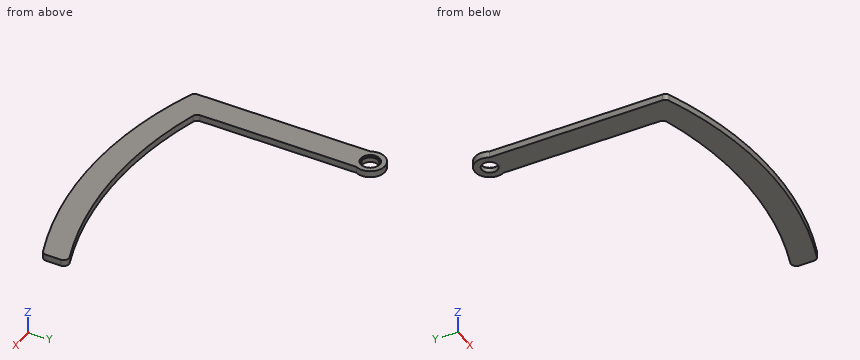
Autodesk Inventor part; units mm, degrees
ref_plane "YZ Plane" through (0, 0, 0) normal (1, 0, 0) x (0, 1, 0)
ref_plane "XZ Plane" through (0, 0, 0) normal (0, 1, 0) x (-1, 0, 0)
ref_plane "XY Plane" through (0, 0, 0) normal (0, 0, 1) x (1, 0, 0)
sketch "スケッチ1" plane through (0, 0, 0) normal (0, 0, 1) x (1, 0, 0)
  line L0 (-5, -38) -> (5, -38)
  line L1 (5, -38) -> (5, 38)
  line L2 (5, 38) -> (-5, 38)
  line L3 (-5, 38) -> (-5, -38)
  line L4 (-5, -38) -> (5, 38) construction
  line L5 (5, -38) -> (-5, 38) construction
  line L6 (-5, -38) -> (100, -38)
  line L7 (100, -38) -> (100, -28)
  line L8 (100, -28) -> (-5, -28)
  line L9 (-5, -28) -> (-5, -38)
  line L10 (47.5, -38) -> (47.5, -48)
  arc A0 (-5, -28) -> (100, -28) centre (47.5, 104.8125) ccw
  arc A1 (-5, -38) -> (100, -38) centre (47.5, 94.8125) ccw
  point P0 (0, 0)
  point P1 (5, -31.5296)
  dimension "d0" = 10
  dimension "d1" = 76
  dimension "d2" = 105
  dimension "d3" = 10
  dimension "d4" = 10
extrude "押し出し1" add sketch "スケッチ1" along normal mid plane 2.5 contours L3 A0 L1 L0 | L0 L6 L10 A1 | L1 A0 L6 | L3 L2 L1 L8 | L8 L1 A0 | L10 L6 A1 | A0 L7 L6 picked at (-0.5654, -28.4196)
sketch "スケッチ2" plane through (0, 0, 1.25) normal (0, 0, 1) x (1, 0, 0)
  line L0 (5, 38) -> (-5, 38)
  line L1 (5, -31.5296) -> (5, 38)
  circle A0 centre (0, 33) radius 3.05
  circle A1 centre (0, 33) radius 3.65
  point P0 (0, 0)
  dimension "d7" = 5
  dimension "d8" = 5
  dimension "d9" = 6.1
  dimension "d10" = 7.3
extrude "押し出し2" cut sketch "スケッチ2" against normal blind 0.6 contours A0 | A1
sketch "スケッチ3" plane through (0, 33, 0.65) normal (0, 0, 1) x (1, 0, 0)
  circle A0 centre (0, 0) radius 3.05
  point P0 (0, -33)
  dimension "d13" = 6.1
extrude "押し出し3" cut sketch "スケッチ3" against normal blind 1.9
sketch "スケッチ6" plane through (0, 0, 1.25) normal (0, 0, 1) x (1, 0, 0)
  circle A0 centre (0, 33) radius 3.65
  line L0 (-5, 38) -> (-5, -38)
  arc A1 (-5, -38) -> (100, -38) centre (47.5, 94.8125) ccw
  line L1 (100, -38) -> (100, -28)
  arc A2 (5, -31.5296) -> (100, -28) centre (47.5, 104.8125) ccw
  line L2 (5, -31.5296) -> (5, 38)
  line L3 (5, 38) -> (-5, 38)
  circle A3 centre (0, 33) radius 5.65
  point P0 (0, 0)
  point P1 (-5, 30.3689)
  point P2 (-5, 35.6311)
  point P3 (-2.6311, 38)
  point P4 (2.6311, 38)
  point P5 (5, 35.6311)
  point P6 (5, 30.3689)
  dimension "d18" = 11.3
extrude "押し出し5" add sketch "スケッチ6" against normal blind 2.5 contours L0 A3 | A3 L3 | L2 A3
sketch "スケッチ7" plane through (0, 0, 1.25) normal (0, 0, 1) x (1, 0, 0)
  circle A0 centre (0, 33) radius 3.65
  line L0 (-5, 38) -> (-5, 35.6311)
  arc A1 (-5, 35.6311) -> (-5, 30.3689) centre (0, 33) ccw
  line L1 (-5, 30.3689) -> (-5, -38)
  arc A2 (-5, -38) -> (100, -38) centre (47.5, 94.8125) ccw
  line L2 (100, -38) -> (100, -28)
  arc A3 (5, -31.5296) -> (100, -28) centre (47.5, 104.8125) ccw
  line L3 (5, -31.5296) -> (5, 30.3689)
  arc A4 (5, 30.3689) -> (5, 35.6311) centre (0, 33) ccw
  line L4 (5, 35.6311) -> (5, 38)
  line L5 (5, 38) -> (2.6311, 38)
  arc A5 (2.6311, 38) -> (-2.6311, 38) centre (0, 33) ccw
  line L6 (-2.6311, 38) -> (-5, 38)
  circle A6 centre (0, 33) radius 5.65
  point P0 (0, 0)
  point P1 (-5, 35.6311)
  point P2 (-2.6311, 38)
  point P3 (2.6311, 38)
  point P4 (5, 35.6311)
extrude "押し出し6" cut sketch "スケッチ7" against normal blind 2.5 contours L6 A6 L0 | L5 L4 A6
fillet "フィレット1" radius 2 4 edges at (-5, -38, 0) (5, -31.5296, 0) (100, -28, 0) (100, -38, 0)
properties part number "指_大"
Read the model definition and answer for the solid it produces. Units are mm, in the model's axes. Round coordinates to 2 decimals unless told otherwise and drop trailing zeros. Write each loop counter-clockwise with the first axis right and the second up, starting at its lowest first coordinate (ties: lowest second). Pieces come first, ordered by that corner, then holes. Notation, with made-up numbers: (67.5, 31) - (105.5, 31) arc R28 cw to (105.5, 49) - close; hole circle Ø1 at (82.25, 47). An arc over 180 degrees is marked (long way). One line per item, written item: value.
Q1. Find section C-C (x = 0). Determine the outline of the cut face in (y, z).
The answers:
outline: (-39.87, -1.25) - (29.95, -1.25) - (29.95, 0.65) - (29.35, 0.65) - (29.35, 1.25) - (-39.87, 1.25) - close; (36.05, -1.25) - (38.65, -1.25) - (38.65, 1.25) - (36.65, 1.25) - (36.65, 0.65) - (36.05, 0.65) - close
Q2. Each of these flat-tipped pins is pushed along its axis until it touches: P1, Ø1.2, axis at y = 8.5, z = -0.5, coming from the -X side; P2, Ø1.2, axis at y = 10.5, z = 0, coming from the +X side; P3, Ø6.5, axis at x = 0, y = 33, coming from the +Z side. Where does it stop, or does it pass through?
The answers:
P1: stops at x = -5
P2: stops at x = 5
P3: stops at z = 0.65
Q3. Find section D-D (y = 9). Determine the outline of the cut face in (x, z), and give its area (3 significant figures).
The answers:
outline: (-5, -1.25) - (5, -1.25) - (5, 1.25) - (-5, 1.25) - close
area: 25.0 mm2
Q4. Find section B-B (y = 33). Determine the outline of the cut face in (x, z), and give its area (3 significant figures).
The answers:
outline: (-5.65, -1.25) - (-3.05, -1.25) - (-3.05, 0.65) - (-3.65, 0.65) - (-3.65, 1.25) - (-5.65, 1.25) - close; (3.05, -1.25) - (5.65, -1.25) - (5.65, 1.25) - (3.65, 1.25) - (3.65, 0.65) - (3.05, 0.65) - close
area: 12.3 mm2
Q5. Straight lines are drawn through the part: line 1 (X direction, y = -12, z = -1); line 2 (Y direction, x = 0, z = 0.9); line 3 (Y direction, x = 2.5, z = -0.55). For each, find the intervals that lie inside material, in ascending order. Write a range as from..to.
The answers:
line 1: x = -5..5
line 2: y = -39.87..29.35, 36.65..38.65
line 3: y = -40.72..31.25, 34.75..38.07
